Could you check a few things on this model? Use its own coordinates, in mm. Face numbers are marked on the shaded views. A direction names the side the tool comes from. Give positions to 0.01 mm unless a question says otherwise; leave off trailing zeros. Loops run counter-clockwise (first coordinate to the right, second up) from the corner with the lowest first, then second, coordinate; pieces in that order, holes last. Notation, with made-up numbers: M 28,18 L 32,18 A21 cw 32,39 Z; hole C -27,35 d5. An arc over 180 degrees is marked long. Use a Markdown table: item, result. Add a question column.
1) If I drill on line 1 along X through (y, z) = (-4.25, -8); line 2 along Z through (x, y) = (2.5, 2.25); line 3 along X through (y, z) = (-6.5, -1), over which ranges is the centre line in solid material (lowest first)? Write a range as [from, to].
2) We'd pull the mould along Z, two halves only. Please class the marked faces 1 and 2: +Z half, -Z half, draft (parallel to the pull), parting line (faces both ways), or undercut.
3) Which directions (+Z, -Z, +X, -X, +Y, -Y) give clear straight access to the entire face, cutting with the end or side of a thin tool? Please do the marked faces 3 and 4.
4) Suppose I cut it at A-A on z = -3. List the corners of the cut face in (x, y) for me.
5) Suppose I cut it at B-B on y = -1. List the corners of the cut face in (x, z) for me, and give its area (3 significant figures).
6) Will this pin go through, and if not, where does the flat tip stop? pin 1 Ø4 at (x, z) = (-6.5, 5.5) entering from +Y (3 decimals).
```python
from build123d import *

# Parameters (mm, degrees)
SKETCH1_W                = 40.2
SKETCH1_H                = 20.2
BOSS_EXTRUDE1_DEPTH      = 7.1
BOSS_EXTRUDE1_DEPTH_BACK = 7.1
FILLET1_R                = 1
SKETCH2_W                = 38.6
SKETCH2_H                = 18.6
CUT_EXTRUDE1_DEPTH       = 1.25
SKETCH3_W                = 37.3
SKETCH3_H                = 17.3
CUT_EXTRUDE2_DEPTH       = 13.95
SKETCH4_W                = 0.3
SKETCH4_H                = 1.2
CUT_EXTRUDE3_DEPTH       = 41.2
LPATTERN1_COUNT          = 6
LPATTERN1_PITCH          = 2.1
MIRROR2_COPY_1_SKETCH_W  = 0.3
MIRROR2_COPY_1_SKETCH_H  = 1.2
MIRROR2_COPY_1_DEPTH     = 41.2
MIRROR2_COPY_2_SKETCH_W  = 0.3
MIRROR2_COPY_2_SKETCH_H  = 1.2
MIRROR2_COPY_2_DEPTH     = 41.2
MIRROR2_COPY_3_SKETCH_W  = 0.3
MIRROR2_COPY_3_SKETCH_H  = 1.2
MIRROR2_COPY_3_DEPTH     = 41.2
MIRROR2_COPY_4_SKETCH_W  = 0.3
MIRROR2_COPY_4_SKETCH_H  = 1.2
MIRROR2_COPY_4_DEPTH     = 41.2
MIRROR2_COPY_5_SKETCH_W  = 0.3
MIRROR2_COPY_5_SKETCH_H  = 1.2
MIRROR2_COPY_5_DEPTH     = 41.2


with BuildPart() as part:
    # Sketch1 → Boss-Extrude1 (new body, two sides)
    with BuildSketch(Plane(origin=(0, 0, 0), x_dir=(1, 0, 0), z_dir=(0, 1, 0))) as boss_extrude1_sk:
        Rectangle(SKETCH1_W, SKETCH1_H)
    extrude(amount=BOSS_EXTRUDE1_DEPTH)
    extrude(boss_extrude1_sk.sketch, amount=-BOSS_EXTRUDE1_DEPTH_BACK)

    # Fillet1
    fillet1_edges = [part.edges().sort_by_distance(p)[0] for p in [
        (-20.1, 0, -10.1),
        (20.1, 0, -10.1),
        (20.1, 0, 10.1),
        (-20.1, 0, 10.1),
    ]]
    fillet(fillet1_edges, radius=FILLET1_R)

    # Sketch2 → Cut-Extrude1 (cut)
    with BuildSketch(Plane(origin=(0, 7.1, 0), x_dir=(1, 0, 0), z_dir=(0, 1, 0))):
        Rectangle(SKETCH2_W, SKETCH2_H)
    cut_extrude1 = extrude(amount=-CUT_EXTRUDE1_DEPTH, mode=Mode.SUBTRACT)

    # Sketch3 → Cut-Extrude2 (cut, through all)
    with BuildSketch(Plane(origin=(0, 5.85, 0), x_dir=(1, 0, 0), z_dir=(0, 1, 0))):
        Rectangle(SKETCH3_W, SKETCH3_H)
    extrude(amount=-CUT_EXTRUDE2_DEPTH, mode=Mode.SUBTRACT)

    # Mirror1: Cut-Extrude1 across plane
    add(cut_extrude1.mirror(Plane.ZX), mode=Mode.SUBTRACT)

    # Sketch4 → Cut-Extrude3 (cut, through all)
    with BuildSketch(Plane(origin=(20.1, 0, 0), x_dir=(0, 0, -1), z_dir=(1, 0, 0))):
        with Locations((-9.95, 5.35)):
            Rectangle(SKETCH4_W, SKETCH4_H)
    cut_extrude3 = extrude(amount=-CUT_EXTRUDE3_DEPTH, mode=Mode.SUBTRACT)

    # LPattern1: Cut-Extrude3 ×6
    with Locations(*[(0, -i * LPATTERN1_PITCH, 0) for i in range(1, LPATTERN1_COUNT)]):
        add(cut_extrude3, mode=Mode.SUBTRACT)

    # Mirror2: Cut-Extrude3 across plane
    add(cut_extrude3.mirror(Plane.XY), mode=Mode.SUBTRACT)

    # Mirror2 copy 1 sketch → Mirror2 copy 1 (cut, through all)
    with BuildSketch(Plane(origin=(20.1, -2.1, 0), x_dir=(0, 0, 1), z_dir=(1, 0, 0))):
        with Locations((-9.95, -5.35)):
            Rectangle(MIRROR2_COPY_1_SKETCH_W, MIRROR2_COPY_1_SKETCH_H)
    extrude(amount=-MIRROR2_COPY_1_DEPTH, mode=Mode.SUBTRACT)

    # Mirror2 copy 2 sketch → Mirror2 copy 2 (cut, through all)
    with BuildSketch(Plane(origin=(20.1, -4.2, 0), x_dir=(0, 0, 1), z_dir=(1, 0, 0))):
        with Locations((-9.95, -5.35)):
            Rectangle(MIRROR2_COPY_2_SKETCH_W, MIRROR2_COPY_2_SKETCH_H)
    extrude(amount=-MIRROR2_COPY_2_DEPTH, mode=Mode.SUBTRACT)

    # Mirror2 copy 3 sketch → Mirror2 copy 3 (cut, through all)
    with BuildSketch(Plane(origin=(20.1, -6.3, 0), x_dir=(0, 0, 1), z_dir=(1, 0, 0))):
        with Locations((-9.95, -5.35)):
            Rectangle(MIRROR2_COPY_3_SKETCH_W, MIRROR2_COPY_3_SKETCH_H)
    extrude(amount=-MIRROR2_COPY_3_DEPTH, mode=Mode.SUBTRACT)

    # Mirror2 copy 4 sketch → Mirror2 copy 4 (cut, through all)
    with BuildSketch(Plane(origin=(20.1, -8.4, 0), x_dir=(0, 0, 1), z_dir=(1, 0, 0))):
        with Locations((-9.95, -5.35)):
            Rectangle(MIRROR2_COPY_4_SKETCH_W, MIRROR2_COPY_4_SKETCH_H)
    extrude(amount=-MIRROR2_COPY_4_DEPTH, mode=Mode.SUBTRACT)

    # Mirror2 copy 5 sketch → Mirror2 copy 5 (cut, through all)
    with BuildSketch(Plane(origin=(20.1, -10.5, 0), x_dir=(0, 0, 1), z_dir=(1, 0, 0))):
        with Locations((-9.95, -5.35)):
            Rectangle(MIRROR2_COPY_5_SKETCH_W, MIRROR2_COPY_5_SKETCH_H)
    extrude(amount=-MIRROR2_COPY_5_DEPTH, mode=Mode.SUBTRACT)


solid = part.part
```
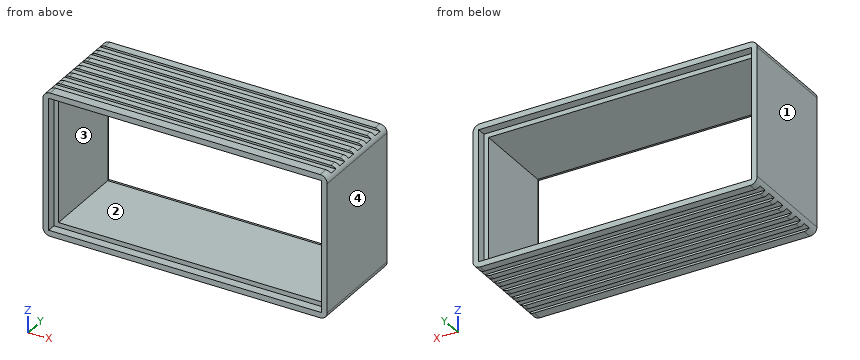
Answer block:
| question | item | result |
|---|---|---|
| 1 | line 1 | x = [-20.1, -18.65], [18.65, 20.1] |
| 1 | line 2 | z = [-10.1, -8.65], [8.65, 10.1] |
| 1 | line 3 | x = [-20.1, -19.3], [19.3, 20.1] |
| 2 | face 1 | draft |
| 2 | face 2 | undercut |
| 3 | face 3 | +Y, -Y |
| 3 | face 4 | +Z, -Z, +X, +Y, -Y |
| 4 | outline | M -20.1,-7.1 L -19.3,-7.1 L -19.3,-5.85 L -18.65,-5.85 L -18.65,5.85 L -19.3,5.85 L -19.3,7.1 L -20.1,7.1 Z; M 18.65,-5.85 L 19.3,-5.85 L 19.3,-7.1 L 20.1,-7.1 L 20.1,7.1 L 19.3,7.1 L 19.3,5.85 L 18.65,5.85 Z |
| 5 | outline | M -20.1,-9.1 A1 ccw -19.81,-9.8 L 19.81,-9.8 A1 ccw 20.1,-9.1 L 20.1,9.1 A1 ccw 19.81,9.8 L -19.81,9.8 A1 ccw -20.1,9.1 Z; hole M -18.65,-8.65 L 18.65,-8.65 L 18.65,8.65 L -18.65,8.65 Z |
| 5 | area | 142 mm^2 |
| 6 | pin 1 | passes through |
